The model under review builds one solid part; all positions refer to its coordinate system, in mm. A direction names the side the tool comes from. Coordinates: 2 decimals unless noted, no trailing zeros. Loops run counter-clockwise (first coordinate to the right, second up) from the corner with the lowest first, then second, coordinate; pieces in that order, holes last. Notation, with made-up numbers: M 74.25,86 L 106.25,86 A20 cw 106.25,115 Z; hole C 29,50 d2. An arc over 180 degrees is marked long. One line per item, written item: value.
```python
from build123d import *

# Parameters (mm, degrees)
SKETCH1_R           = 7
SKETCH1_W           = 22.5
SKETCH1_H           = 12.2
BOSS_EXTRUDE1_DEPTH = 8.55
SKETCH2_W           = 34
SKETCH2_H           = 12.2
CUT_EXTRUDE1_DEPTH  = 4.55
SKETCH3_R           = 9
CUT_EXTRUDE2_DEPTH  = 2
SKETCH4_R           = 8
CUT_EXTRUDE3_DEPTH  = 3.9
CHAMFER1_SIZE       = 0.5
BOSS_EXTRUDE2_DEPTH = 8
SKETCH6_R           = 1.6
CUT_EXTRUDE4_DEPTH  = 5
CUT_EXTRUDE5_REACH  = 82.824
SKETCH7_R           = 3
SKETCH8_W           = 8
SKETCH8_H           = 16.5
BOSS_EXTRUDE3_DEPTH = 8
CHAMFER2_SIZE       = 8


# Read off the part's stored shape, not the designer's step: Mirror3
with BuildPart() as part:
    # Sketch1 → Boss-Extrude1 (new body)
    with BuildSketch(Plane(origin=(0, 0, 0), x_dir=(1, 0, 0), z_dir=(0, 1, 0))):
        with BuildLine():
            Line((-25, 19), (-11.454535097, 50.00436067))
            ThreePointArc((-11.454535097, 50.00436067), (0, 57.5), (11.454535097, 50.00436067))
            Line((11.454535097, 50.00436067), (25, 19))
            Line((25, 19), (25, -19))
            Line((25, -19), (-25, -19))
            Line((-25, -19), (-25, 19))
        make_face()
        with Locations(Location((0, 45, 0), (0, 0, 270))):
            Circle(SKETCH1_R, mode=Mode.SUBTRACT)
        with Locations((0, 7.9)):
            Rectangle(SKETCH1_W, SKETCH1_H, mode=Mode.SUBTRACT)
    extrude(amount=BOSS_EXTRUDE1_DEPTH)

    # Sketch2 → Cut-Extrude1 (cut)
    with BuildSketch(Plane(origin=(0, 8.55, 0), x_dir=(1, 0, 0), z_dir=(0, 1, 0))):
        with Locations((0, 7.9)):
            Rectangle(SKETCH2_W, SKETCH2_H)
    extrude(amount=-CUT_EXTRUDE1_DEPTH, mode=Mode.SUBTRACT)

    # Sketch3 → Cut-Extrude2 (cut)
    with BuildSketch(Plane(origin=(0, 8.55, 0), x_dir=(1, 0, 0), z_dir=(0, 1, 0))):
        with Locations(Location((0, 45, 0), (0, 0, 270))):
            Circle(SKETCH3_R)
    extrude(amount=-CUT_EXTRUDE2_DEPTH, mode=Mode.SUBTRACT)

    # Sketch4 → Cut-Extrude3 (cut)
    with BuildSketch(Plane(origin=(0, 6.55, 0), x_dir=(1, 0, 0), z_dir=(0, 1, 0))):
        with Locations(Location((0, 45, 0), (0, 0, 270))):
            Circle(SKETCH4_R)
    extrude(amount=-CUT_EXTRUDE3_DEPTH, mode=Mode.SUBTRACT)

    # Chamfer1
    chamfer1_edges = [part.edges().sort_by_distance(p)[0] for p in [
        (0, 0, -52),
    ]]
    chamfer(chamfer1_edges, length=CHAMFER1_SIZE)

    # Sketch5 → Boss-Extrude2 (add)
    with BuildSketch(Plane.ZY.offset(25)):
        Polygon((19, 8.55), (19, 28.2), (11, 28.2), (-14, 8.55), align=None)
    extrude(amount=-BOSS_EXTRUDE2_DEPTH)

    # Sketch6 → Cut-Extrude4 (cut)
    with BuildSketch(Plane.XY.offset(19)):
        with Locations((-21, 21.2)):
            Circle(SKETCH6_R)
    cut_extrude4 = extrude(amount=-CUT_EXTRUDE4_DEPTH, mode=Mode.SUBTRACT)

    # Cut-Extrude5: up to this plane
    cut_extrude5_end = Plane(origin=(-17, 28.2, 11), z_dir=(0, 0.7862091997273701, -0.617960430985713))
    # Sketch7 → Cut-Extrude5 (cut, up to the surface)
    with BuildSketch(Plane.XY.offset(14), mode=Mode.PRIVATE) as cut_extrude5_sk1:
        with Locations((-21, 21.2)):
            Circle(SKETCH7_R)
    cut_extrude5_tool1 = split(extrude(cut_extrude5_sk1.sketch, amount=-CUT_EXTRUDE5_REACH, mode=Mode.PRIVATE), bisect_by=cut_extrude5_end, keep=Keep.BOTH, mode=Mode.PRIVATE)
    cut_extrude5 = cut_extrude5_tool1.solids().sort_by_distance((-21, 21.2, 14))[0]
    add(cut_extrude5, mode=Mode.SUBTRACT)

    # Sketch8 → Boss-Extrude3 (add)
    with BuildSketch(Plane.ZY.offset(25)):
        with Locations((15, -8.25)):
            Rectangle(SKETCH8_W, SKETCH8_H)
    extrude(amount=-BOSS_EXTRUDE3_DEPTH)

    # Chamfer2
    chamfer2_edges = [part.edges().sort_by_distance(p)[0] for p in [
        (-21, 0, 11),
    ]]
    chamfer(chamfer2_edges, length=CHAMFER2_SIZE)

    # Mirror2: Cut-Extrude4, Cut-Extrude5 across plane
    add(cut_extrude4.mirror(Plane.ZX.offset(5.85)), mode=Mode.SUBTRACT)
    add(cut_extrude5.mirror(Plane.ZX.offset(5.85)), mode=Mode.SUBTRACT)

    # Mirror3: part across plane


with BuildPart() as part_1:
    add(part.part)
    add(part.part.mirror(Plane(origin=(0, 0, 0), x_dir=(0, 0, 1), z_dir=(1, 0, 0))))


solid = part_1.part
```
(1) Add section A-A on y = 1.5. State the section outline as (x, z) points, then the cut area to 3 significant figures.
Checks:
outline: M -25,-19 L -11.45,-50 A12.5 ccw 11.45,-50 L 25,-19 L 25,19 L -25,19 Z; hole M -11.25,-14 L 11.25,-14 L 11.25,-1.8 L -11.25,-1.8 Z; hole C 0,-45 d14
area: 2,730 mm^2
(2) To check wall thickness, follow L1, parallel to Y at x = -21, z = 15.2; L2, parallel to X at y = -9.5, z = 15.25; L3, parallel to Z at x = 0, y = 1.3. State the ranges of each line that lie inside material, in increasing order. Write a range as [from, to].
Checks:
L1: [-16.5, -11.1], [-7.9, 19.6], [22.8, 28.2]
L2: [-25, -22.6], [-19.4, -17], [17, 19.4], [22.6, 25]
L3: [-57.5, -52], [-38, -14], [-1.8, 19]
(3) Add section D-D on y = -3.5. State the section outline as (x, z) points.
Checks:
outline: M -25,6.5 L -17,6.5 L -17,19 L -25,19 Z; M 17,6.5 L 25,6.5 L 25,19 L 17,19 Z
(4) Tool access review of faces 4 (the face through (17, -6, 14)), 5 (the face through (0, 8.55, 8)), 6 (the face through (0, 0, -20)), 7 (the face through (-6, 2.65, -41)): name each direction out of +Z, -Z, +X, -X, +Y, -Y from which nothing blocks a thin tool from reaching the whole face with its end or side.
Checks:
face 4: +Z, -Z, -Y
face 5: +Z, -Z, +Y
face 6: -Z, -Y
face 7: +Y
(5) Draft analysis for pull direction Z (two halves, no side actions). For faces 1 (the face through (-21.65, 18.27, 8)), 2 (the face through (-18.32, 4.22, -34.29)), 3 (the face through (-14, 4, -8)), state which applies: pulls with the +Z half, pulls with the -Z half, needs draft (parallel to the pull), parting line crosses it, or undercut.
Checks:
face 1: needs draft
face 2: pulls with the -Z half
face 3: undercut
(6) Add section B-B on z = -9. State the section outline as (x, y) points, then the cut area to 3 significant figures.
Checks:
outline: M -25,0 L -11.25,0 L -11.25,4 L -17,4 L -17,12.48 L -25,12.48 Z; M 11.25,0 L 25,0 L 25,12.48 L 17,12.48 L 17,4 L 11.25,4 Z
area: 246 mm^2
(7) Add section C-C on x = 21. State the section outline as (y, z) points.
Checks:
outline: M -16.5,11 L -12.5,11 L -12.5,14 L -11.1,14 L -11.1,19 L -16.5,19 Z; M -7.9,14 L -6.5,14 L -6.5,9.5 L 0,3 L 0,-28.16 L 8.55,-28.16 L 8.55,-14 L 18.2,-1.72 L 18.2,14 L 19.6,14 L 19.6,19 L -7.9,19 Z; M 22.8,14 L 24.2,14 L 24.2,5.91 L 28.2,11 L 28.2,19 L 22.8,19 Z
(8) Insertion check: pin 1 Ø7 at (x, y) = (-21, 21.2) entering from -Z; pin 2 Ø3.5 at (x, y) = (21, -9.5) entering from +Z; pin 3 Ø21 at (x, z) = (0, -45) entering from +Y; pin 4 Ø3 at (x, z) = (-14.5, -5.5) entering from +Y. Each pin has a flat end and moves straight along its axis. Give the tip position at first contact, or say it passes through.
Checks:
pin 1: z = -2.36
pin 2: z = 19
pin 3: y = 8.55
pin 4: y = 4
